from build123d import *

# Parameters (mm, degrees)
SKETCH204_R             = 2.25
PAD094_DEPTH            = 10
POCKET084_DEPTH         = 7
POCKET085_DEPTH         = 3.5
SKETCH213_R             = 2.25
POCKET086_DEPTH         = 10
SKETCH214_R             = 3.75
POCKET087_DEPTH         = 8
BODY025_PLACEMENT_ANGLE = 180


with BuildPart() as part:
    # Sketch204 → Pad094 (new body)
    with BuildSketch(Plane.XY):
        with BuildLine():
            ThreePointArc((5, 18), (0, 43), (-5, 18))
            Line((-5, 18), (-5, -18))
            ThreePointArc((-5, -18), (0, -43), (5, -18))
            Line((5, 18), (5, -18))
        make_face()
        with Locations((0, 13)):
            Circle(SKETCH204_R, mode=Mode.SUBTRACT)
        with Locations((0, -13)):
            Circle(SKETCH204_R, mode=Mode.SUBTRACT)
    extrude(amount=PAD094_DEPTH)

    # Sketch211 → Pocket084 (cut)
    with BuildSketch(Plane.XY):
        with BuildLine():
            Line((-5, 13.000202), (-5, -12.999798))
            ThreePointArc((5, -12.999798), (0, -7.999799), (-5, -12.999798))
            Line((5, -12.999798), (5, 13.000202))
            ThreePointArc((-5, 13.000202), (0, 8.000186), (5, 13.000202))
        make_face()
    extrude(amount=POCKET084_DEPTH, mode=Mode.SUBTRACT)

    # Sketch212 → Pocket085 (cut, symmetric)
    with BuildSketch(Plane.XY):
        Polygon((0, -21), (-3.464102, -23), (-3.464102, -27), (0, -29), (3.464102, -27), (3.464102, -23), align=None)
        Polygon((0, 21), (3.464102, 23), (3.464102, 27), (0, 29), (-3.464102, 27), (-3.464102, 23), align=None)
    extrude(amount=POCKET085_DEPTH, both=True, mode=Mode.SUBTRACT)

    # Sketch213 → Pocket086 (cut)
    with BuildSketch(Plane.XY):
        with Locations((0, 25)):
            Circle(SKETCH213_R)
        with Locations((0, -25)):
            Circle(SKETCH213_R)
    extrude(amount=POCKET086_DEPTH, mode=Mode.SUBTRACT)

    # Sketch214 (on Face5 of Pocket086) → Pocket087 (cut)
    with BuildSketch(Plane.XY.offset(10)):
        with Locations((0, 13)):
            Circle(SKETCH214_R)
        with Locations((0, -13)):
            Circle(SKETCH214_R)
    extrude(amount=-POCKET087_DEPTH, mode=Mode.SUBTRACT)


with BuildPart() as part_1:
    # Body025 placement: moved
    add(part.part.moved(Location((0, 91, -15))).rotate(Axis((0, 91, -15), (0, 1, 0)), BODY025_PLACEMENT_ANGLE))


solid = part_1.part
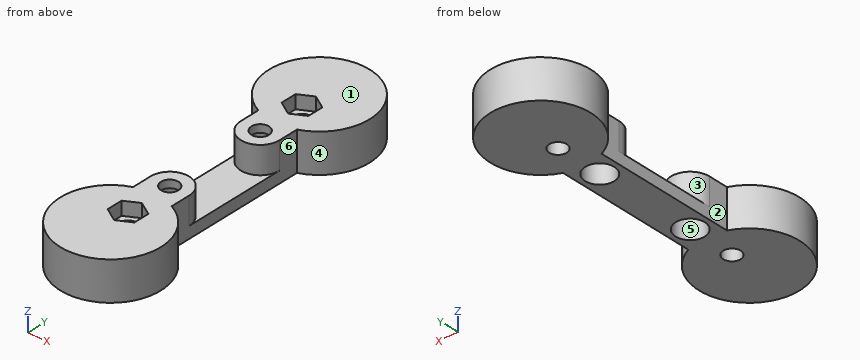
Design review of the part built by this model. Coordinates are the model's own, in mm. Face numbers are marked on the shaded views. A direction names the side the tool comes from. Coordinates: 2 decimals unless noted, no trailing zeros. Write each loop counter-clockwise with the first axis right and the second up, starting at its lowest first coordinate (ties: lowest second). Pieces come first, ordered by that corner, then holes. Notation, with made-up numbers: (-3.75, 79) - (50.25, 79) arc R11 ccw to (50.25, 99) - close; hole circle Ø6 at (-20.5, 6). An arc over 180 degrees is marked (long way). One line per item, written item: value.
1) Mouldability with a two-part tool opening along Y and no side actions: class the marked faces 1 and 2 as +Y half, -Y half, draft (parallel to the pull), parting line (faces both ways), or undercut.
Answer sheet:
face 1: draft
face 2: undercut
2) Add section C-C (x = 7.75). State the section outline as (y, z) points.
Answer sheet:
outline: (50.56, -25) - (71.44, -25) - (71.44, -15) - (50.56, -15) - close; (110.56, -25) - (131.44, -25) - (131.44, -15) - (110.56, -15) - close
3) For the marked faces 3, 4, 5 and 6, list the 3-axis set-ups (+Z, -Z, +X, -X, +Y, -Y) from which the entire face can be reached by the end or side of a thin tool; tool diameter is ignored.
Answer sheet:
face 3: +Z
face 4: +Z, -Z
face 5: -Z
face 6: +Z, -Z, +X
4) Insertion check: pin 1 (4 mm diameter, centred on y = 66, z = -16, fed in from +X); pin 2 (3.5 mm diameter, centred on x = 0, y = 78, fed in from -Z); pin 3 (6 mm diameter, centred on x = 0, y = 104, fed in from -Z); pin 4 (2 mm diameter, centred on x = 1, y = 67.5, fed in from +Z). Each pin has a flat end and moves straight along its axis. Give the tip position at first contact, or say it passes through.
Answer sheet:
pin 1: stops at x = 12.65
pin 2: passes through
pin 3: stops at z = -17
pin 4: stops at z = -18.5
5) Add section D-D (y = 116). State the section outline as (x, z) points, plus the area to 3 significant figures.
Answer sheet:
outline: (-12, -25) - (-2.25, -25) - (-2.25, -18.5) - (-3.46, -18.5) - (-3.46, -15) - (-12, -15) - close; (2.25, -25) - (12, -25) - (12, -15) - (3.46, -15) - (3.46, -18.5) - (2.25, -18.5) - close
area: 187 mm2
6) To check wall thickness, follow probe 1 along X at (y, z) = (78, -16.45); probe 2 along X at (y, z) = (66, -20.75); probe 3 along Z at (x, y) = (-4, 92). State the ranges of each line that lie inside material, in increasing order.
Answer sheet:
probe 1: x = -5 to -2.25, 2.25 to 5
probe 2: x = -12 to -2.25, 2.25 to 12
probe 3: z = -25 to -22
7) Add section A-A (z = -16.25). State the section outline as (x, y) points.
Answer sheet:
outline: (-5, 73) arc R13 ccw (long way) to (5, 73) - (5, 78) arc R5 ccw to (-5, 78) - close; (-5, 104) arc R5 ccw to (5, 104) - (5, 109) arc R13 ccw (long way) to (-5, 109) - close; hole (-3.46, 64) - (0, 62) - (3.46, 64) - (3.46, 68) - (0, 70) - (-3.46, 68) - close; hole (-3.46, 114) - (0, 112) - (3.46, 114) - (3.46, 118) - (0, 120) - (-3.46, 118) - close; hole circle Ø4.5 at (0, 78); hole circle Ø4.5 at (0, 104)
8) Add section B-B (z = -22.75). State the section outline as (x, y) points.
Answer sheet:
outline: (-5, 73) arc R13 ccw (long way) to (5, 73) - (5, 109) arc R13 ccw (long way) to (-5, 109) - close; hole circle Ø7.5 at (0, 78); hole circle Ø7.5 at (0, 104); hole circle Ø4.5 at (0, 66); hole circle Ø4.5 at (0, 116)
